from build123d import *

# Parameters (mm, degrees)
F0_R     = 6.625
F0_R_2   = 4
F1_DEPTH = 1.5
F2_DEPTH = 3
F3_T     = -1


with BuildPart() as f1:
    # F0 (on Top) → F1 (new body)
    with BuildSketch(Plane.XY):
        Circle(F0_R)
        Circle(F0_R_2, mode=Mode.SUBTRACT)
        Circle(F0_R_2)
    extrude(amount=F1_DEPTH)

    # F0 (on Top) → F2 (join)
    with BuildSketch(Plane.XY):
        Circle(F0_R_2)
    extrude(amount=-F2_DEPTH)

    # F3
    f3_openings = [f1.faces().sort_by_distance(p)[0] for p in [
        (0, 0, -3),
    ]]
    offset(amount=F3_T, openings=f3_openings, kind=Kind.INTERSECTION)


solid = f1.part
Input: part model. Units: mm. Frame: model coordinates. A direction names the side the tool comes from. Coordinates: 2 decimals unless noted, no trailing zeros. Write each loop counter-clockwise with the first axis right and the second up, starting at its lowest first coordinate (ties: lowest second). Pieces come first, ordered by that corner, then holes. Notation, with made-up numbers: M 54,11.25 L 74,11.25 A23 ccw 74,45.25 Z; hole C 71,54.5 d2. An arc over 180 degrees is marked long. Answer as a JSON object with one key per item and string values. Group by question number.
(1) Set-up query: faces 1 (the face through (3, -3, 0)), 2 (the face through (1, 3, -3)). Return all of +Z, -Z, +X, -X, +Y, -Y with unobstructed straight access to the full face (end or side cutting, diameter ignored); none if empty.
(2) Section A-A on x = 0. Output: boundary loops of the cut face in (y, z) (3 decimals).
(3) Mould query, pull axis Y, two halves, no side actions, for faces 3 (the face through (0, 0, 1.5)), 4 (the face through (-0.867, -3.905, -1.479)), 5 (the face through (-3, 0, -1)). Classes: pulls with the +Y half, pulls with the -Y half, needs draft (parallel to the pull), parting line crosses it, or undercut.
(4) Section C-C on z = -1.3. Output: boundary loops of the cut face in (x, y).
(5) Section D-D on z = 0.75. Output: boundary loops of the cut face in (x, y) (3 decimals).
(6) Ray query, line 1 along Y through (x, z) = (0, -1.85); line 2 along Z through (x, y) = (6.25, 0.25); line 3 along Z through (x, y) = (-2.75, 0.25). Return the intervals inside material, ascending. Write a range as [from, to].
(7) Contact query for flat-ended pins moving along their axis: P1, Ø3.5, axis at x = 0, y = 0, coming from the -Z side; P2, Ø1.5, axis at x = 2, z = -0.5, coming from the -Y side. Output: stop coordinate, or through.
Result set:
{
 "1": {"face 1": "-Z", "face 2": "-Z, +X, -X, +Y, -Y"},
 "2": {"outline": "M -6.625,0 L -4,0 L -4,-3 L -3,-3 L -3,0.5 L 3,0.5 L 3,-3 L 4,-3 L 4,0 L 6.625,0 L 6.625,1.5 L -6.625,1.5 Z"},
 "3": {"face 3": "needs draft", "face 4": "parting line crosses it", "face 5": "undercut"},
 "4": {"outline": "C 0,0 d8; hole C 0,0 d6"},
 "5": {"outline": "C 0,0 d13.25"},
 "6": {"line 1": "y = [-4, -3], [3, 4]", "line 2": "z = [0, 1.5]", "line 3": "z = [0.5, 1.5]"},
 "7": {"P1": "stops at z = 0.5", "P2": "stops at y = -6.47"}
}
